Input: dimensioned drawing with shaded views. Units: mm. Origin: part minimum x, y, z. Round coordinates to 2 decimals unless told otherwise and drop trailing zeros. Loops run counter-clockwise (first coordinate to the right, second up) from the corner with the lowest first, then second, coordinate; pieces in that order, holes last. Notation, with made-up numbers: (13, -35) - (33, -35) arc R23 ccw to (33, -14) - close; hole circle Ø10 at (-26, -14.75). An arc over 180 degrees is marked (long way). Answer as a JSON object with one key per item and string values. Group by question number.
Item 1: Section C-C (z = 13.25). Return the cut outline in (x, y), plus the area to 3 significant figures.
Item 2: Section D-D (z = 24.25). Return the cut outline in (x, y).
Item 3: Section B-B (y = 10). Return the cut outline in (x, z).
Item 4: First-contact query: pin 1 (9 mm diameter, centred on y = 10, z = 15, fed in from -X). Flat tip, straight axial feed; report the tip coordinate or a pass-through.
Item 5: Draft query along Z for the marked faces 1, 2 and 3. Return one class per face: released by +Z, released by -Z, zero draft, split by the parting line, or undercut.
Item 6: Section A-A (x = 20). Return the cut outline in (y, z).
Item 7: Line query: line 1 (Y direction, x = 20, z = 15.25); line 2 (X direction, y = 25, z = 10.25); line 3 (Y direction, x = 27, z = 15). Output: solid intervals per line, ascending.
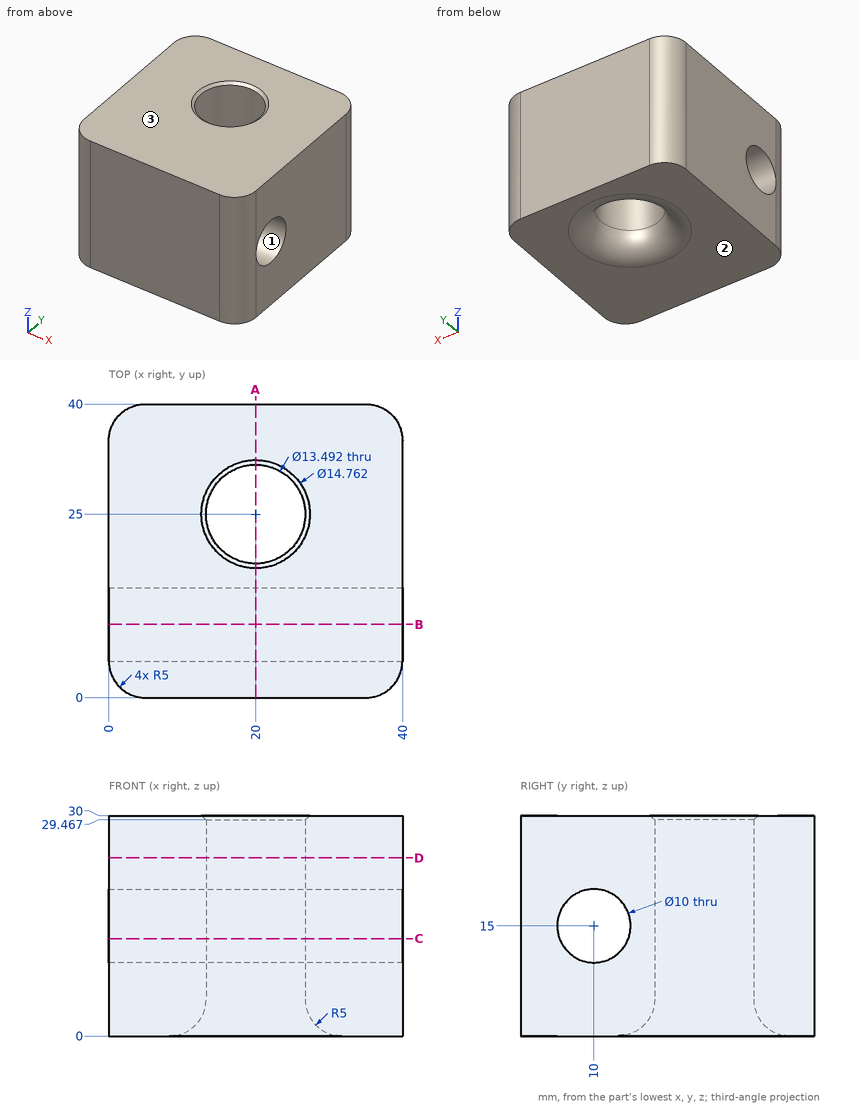
Values:
{
 "1": {"outline": "(0, 5) arc R5 ccw to (5, 0) - (35, 0) arc R5 ccw to (40, 5) - (40, 5.32) - (0, 5.32) - close; (0, 14.68) - (40, 14.68) - (40, 35) arc R5 ccw to (35, 40) - (5, 40) arc R5 ccw to (0, 35) - close; hole circle Ø13.49 at (20, 25)", "area": "1,060 mm^2"},
 "2": {"outline": "(0, 5) arc R5 ccw to (5, 0) - (35, 0) arc R5 ccw to (40, 5) - (40, 35) arc R5 ccw to (35, 40) - (5, 40) arc R5 ccw to (0, 35) - close; hole circle Ø13.49 at (20, 25)"},
 "3": {"outline": "(0, 0) - (40, 0) - (40, 10) - (0, 10) - close; (0, 20) - (40, 20) - (40, 30) - (0, 30) - close"},
 "4": {"pin 1": "passes through"},
 "5": {"face 1": "undercut", "face 2": "released by -Z", "face 3": "released by +Z"},
 "6": {"outline": "(0, 0) - (13.25, 0) arc R5 ccw to (18.25, 5) - (18.25, 29.47) - (17.62, 30) - (0, 30) - close; (31.75, 5) arc R5 ccw to (36.75, 0) - (40, 0) - (40, 30) - (32.38, 30) - (31.75, 29.47) - close; hole circle Ø10 at (10, 15)"},
 "7": {"line 1": "y = 0 to 5.01, 14.99 to 18.25, 31.75 to 40", "line 2": "x = 0 to 13.25, 26.75 to 40", "line 3": "y = 0 to 5, 15 to 40"}
}
